Here's how the part is built. I have some questions about the finished solid (model axes, mm). Face numbers are marked on the shaded views. A direction names the side the tool comes from. Give positions to 0.01 mm unless a question says otherwise; leave off trailing zeros. Write each loop counter-clockwise with the first axis right and the second up, starting at its lowest first coordinate (ties: lowest second). Pieces come first, ordered by that corner, then holes. Notation, with made-up numbers: (-24, -17.75) - (12, -17.75) arc R16 ccw to (12, -6.75) - close; hole circle Ø3 at (50.5, -30.75). An arc over 180 degrees is marked (long way). Write each question's results on one line, items separated by ' | '. Start each with the question number.
Item 1: Suppose I cut it at A-A on y = -1.25. List the corners of the cut face in (x, z) for me (3 decimals).
Item 2: Please list where these lines run through material, in increasing order: line 1 along X through (y, z) = (-1, 0.55); line 2 along Y through (x, z) = (4.5, 4.25); line 3 along Y through (x, z) = (-9, 2.55).
Item 3: Suppose I cut it at D-D on y = -4. List the corners of the cut face in (x, z) for me (3 decimals).
Item 4: We'd pull the mould along X, two halves only. Please class the marked faces 3, 4 and 5: +X half, -X half, draft (parallel to the pull), parting line (faces both ways), or undercut.
Item 5: Suppose I cut it at B-B on z = 3.8. List the corners of the cut face in (x, y) for me.
Item 6: Suppose I cut it at C-C on x = 5. List the corners of the cut face in (y, z) for me (3 decimals), then the cut area to 3 significant figures.
Item 7: Which directions (+Z, -Z, +X, -X, +Y, -Y) give clear straight access to the entire face, cutting with the end or side of a thin tool? Please do the marked faces 1 and 2.
Autodesk Inventor part; units mm, degrees
ref_plane "YZ Plane" through (0, 0, 0) normal (1, 0, 0) x (0, 1, 0)
ref_plane "XZ Plane" through (0, 0, 0) normal (0, 1, 0) x (-1, 0, 0)
ref_plane "XY Plane" through (0, 0, 0) normal (0, 0, 1) x (1, 0, 0)
sketch "Sketch1" plane through (0, 0, 0) normal (0, 0, 1) x (1, 0, 0)
  line L0 (-10, 5) -> (10, 5)
  line L1 (10, 5) -> (10, -5)
  line L2 (10, -5) -> (-10, -5)
  line L3 (-10, -5) -> (-10, 5)
  line L4 (-5.5, 2) -> (-4, 2)
  line L5 (-4, 2) -> (-4, -2)
  line L6 (-4, -2) -> (-5.5, -2)
  line L7 (-5.5, -2) -> (-5.5, 2)
  line L8 (5.5, 2) -> (4, 2)
  line L9 (4, 2) -> (4, -2)
  line L10 (4, -2) -> (5.5, -2)
  line L11 (5.5, -2) -> (5.5, 2)
  line L12 (-4, 0) -> (4, 0)
  point P0 (0, 0)
  point P1 (-10, 0)
  point P2 (0, 5)
  point P3 (0, 0)
  dimension "d0" = 20
  dimension "d2" = 10
  dimension "d3" = 8
  dimension "d4" = 1.5
  dimension "d5" = 4
extrude "Extrusion1" add sketch "Sketch1" along normal blind 5.715
fillet "Fillet1" radius 2 4 edges at (-10, 5, 2.8575) (10, 5, 2.8575) (10, -5, 2.8575) (-10, -5, 2.8575)
properties part number "RETAINER"
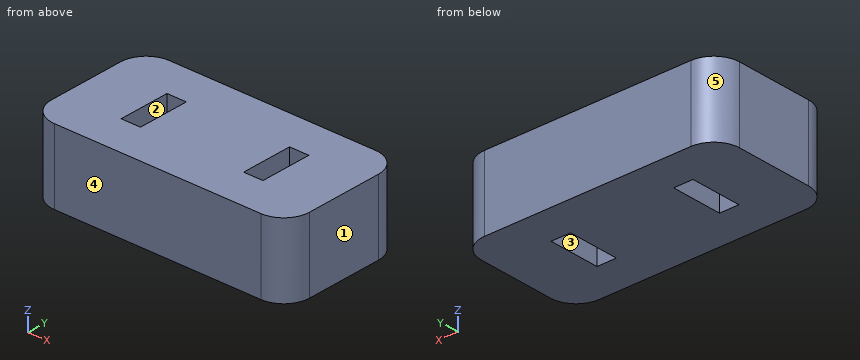
Checked values:
1) outline: (-10, 0) - (-5.5, 0) - (-5.5, 5.715) - (-10, 5.715) - close; (-4, 0) - (4, 0) - (4, 5.715) - (-4, 5.715) - close; (5.5, 0) - (10, 0) - (10, 5.715) - (5.5, 5.715) - close
2) line 1: x = -10 to -5.5, -4 to 4, 5.5 to 10 | line 2: y = -5 to -2, 2 to 5 | line 3: y = -4.73 to 4.73
3) outline: (-9.732, 0) - (9.732, 0) - (9.732, 5.715) - (-9.732, 5.715) - close
4) face 3: undercut | face 4: draft | face 5: -X half
5) outline: (-10, -3) arc R2 ccw to (-8, -5) - (8, -5) arc R2 ccw to (10, -3) - (10, 3) arc R2 ccw to (8, 5) - (-8, 5) arc R2 ccw to (-10, 3) - close; hole (-5.5, -2) - (-4, -2) - (-4, 2) - (-5.5, 2) - close; hole (4, -2) - (5.5, -2) - (5.5, 2) - (4, 2) - close
6) outline: (-5, 0) - (-2, 0) - (-2, 5.715) - (-5, 5.715) - close; (2, 0) - (5, 0) - (5, 5.715) - (2, 5.715) - close | area: 34.3 mm^2
7) face 1: +Z, -Z, +X, +Y, -Y | face 2: +Z, -Z
